```python
from build123d import *

# Parameters (mm, degrees)
SKETCH1_W           = 239
SKETCH1_H           = 85.4
BOSS_EXTRUDE1_DEPTH = 5
SKETCH2_R           = 1.58
CUT_EXTRUDE1_DEPTH  = 254.848695092
CUT_EXTRUDE2_DEPTH  = 254.848695092
SKETCH4_R           = 2.5
SKETCH4_W           = 50
SKETCH4_H           = 15
SKETCH4_W_2         = 19.5
SKETCH4_H_2         = 14
CUT_EXTRUDE3_DEPTH  = 254.848695092
SKETCH5_W           = 5
SKETCH5_H           = 85.4
BOSS_EXTRUDE2_DEPTH = 3


with BuildPart() as part:
    # Sketch1 → Boss-Extrude1 (new body)
    with BuildSketch(Plane.XY):
        with Locations((119.5, 42.7)):
            Rectangle(SKETCH1_W, SKETCH1_H)
    extrude(amount=BOSS_EXTRUDE1_DEPTH)

    # Sketch2 → Cut-Extrude1 (cut, through all)
    with BuildSketch(Plane.XY.offset(5)):
        with Locations((30, 30)):
            Circle(SKETCH2_R)
        with Locations((54.99, 30)):
            Circle(SKETCH2_R)
        with Locations((94.99, 30)):
            Circle(SKETCH2_R)
        with Locations((70, 30)):
            Circle(SKETCH2_R)
        with Locations((134.99, 30)):
            Circle(SKETCH2_R)
        with Locations((110, 30)):
            Circle(SKETCH2_R)
        with Locations((94.99, 50)):
            Circle(SKETCH2_R)
        with Locations((70, 50)):
            Circle(SKETCH2_R)
        with Locations((134.99, 50)):
            Circle(SKETCH2_R)
        with Locations((110, 50)):
            Circle(SKETCH2_R)
        with Locations((94.99, 70)):
            Circle(SKETCH2_R)
        with Locations((70, 70)):
            Circle(SKETCH2_R)
        with Locations((134.99, 70)):
            Circle(SKETCH2_R)
        with Locations((110, 70)):
            Circle(SKETCH2_R)
        with Locations((54.99, 50)):
            Circle(SKETCH2_R)
        with Locations((30, 50)):
            Circle(SKETCH2_R)
        with Locations((54.99, 70)):
            Circle(SKETCH2_R)
        with Locations((30, 70)):
            Circle(SKETCH2_R)
    extrude(amount=-CUT_EXTRUDE1_DEPTH, mode=Mode.SUBTRACT)

    # Sketch3 → Cut-Extrude2 (cut, through all)
    with BuildSketch(Plane.XY.offset(5)):
        with BuildLine():
            Line((31.5267187, 33.043828447), (32.799320889, 24.771914224))
            ThreePointArc((32.799320889, 24.771914224), (33.305182132, 23.861551788), (34.281878435, 23.5))
            Line((34.281878435, 23.5), (50.708121565, 23.5))
            ThreePointArc((50.708121565, 23.5), (51.684817868, 23.861551788), (52.190679111, 24.771914224))
            Line((52.190679111, 24.771914224), (53.4632813, 33.043828447))
            ThreePointArc((53.4632813, 33.043828447), (52.775062631, 35.453392605), (50.498166207, 36.5))
            Line((50.498166207, 36.5), (34.491833793, 36.5))
            ThreePointArc((34.491833793, 36.5), (32.214937369, 35.453392605), (31.5267187, 33.043828447))
        make_face()
        with BuildLine():
            Line((71.5267187, 33.043828447), (72.799320889, 24.771914224))
            ThreePointArc((72.799320889, 24.771914224), (73.305182132, 23.861551788), (74.281878435, 23.5))
            Line((74.281878435, 23.5), (90.708121565, 23.5))
            ThreePointArc((90.708121565, 23.5), (91.684817868, 23.861551788), (92.190679111, 24.771914224))
            Line((92.190679111, 24.771914224), (93.4632813, 33.043828447))
            ThreePointArc((93.4632813, 33.043828447), (92.775062631, 35.453392605), (90.498166207, 36.5))
            Line((90.498166207, 36.5), (74.491833793, 36.5))
            ThreePointArc((74.491833793, 36.5), (72.214937369, 35.453392605), (71.5267187, 33.043828447))
        make_face()
        with BuildLine():
            Line((111.5267187, 33.043828447), (112.799320889, 24.771914224))
            ThreePointArc((112.799320889, 24.771914224), (113.305182132, 23.861551788), (114.281878435, 23.5))
            Line((114.281878435, 23.5), (130.708121565, 23.5))
            ThreePointArc((130.708121565, 23.5), (131.684817868, 23.861551788), (132.190679111, 24.771914224))
            Line((132.190679111, 24.771914224), (133.4632813, 33.043828447))
            ThreePointArc((133.4632813, 33.043828447), (132.775062631, 35.453392605), (130.498166207, 36.5))
            Line((130.498166207, 36.5), (114.491833793, 36.5))
            ThreePointArc((114.491833793, 36.5), (112.214937369, 35.453392605), (111.5267187, 33.043828447))
        make_face()
        with BuildLine():
            Line((71.5267187, 53.043828447), (72.799320889, 44.771914224))
            ThreePointArc((72.799320889, 44.771914224), (73.305182132, 43.861551788), (74.281878435, 43.5))
            Line((74.281878435, 43.5), (90.708121565, 43.5))
            ThreePointArc((90.708121565, 43.5), (91.684817868, 43.861551788), (92.190679111, 44.771914224))
            Line((92.190679111, 44.771914224), (93.4632813, 53.043828447))
            ThreePointArc((93.4632813, 53.043828447), (92.775062631, 55.453392605), (90.498166207, 56.5))
            Line((90.498166207, 56.5), (74.491833793, 56.5))
            ThreePointArc((74.491833793, 56.5), (72.214937369, 55.453392605), (71.5267187, 53.043828447))
        make_face()
        with BuildLine():
            Line((111.5267187, 53.043828447), (112.799320889, 44.771914224))
            ThreePointArc((112.799320889, 44.771914224), (113.305182132, 43.861551788), (114.281878435, 43.5))
            Line((114.281878435, 43.5), (130.708121565, 43.5))
            ThreePointArc((130.708121565, 43.5), (131.684817868, 43.861551788), (132.190679111, 44.771914224))
            Line((132.190679111, 44.771914224), (133.4632813, 53.043828447))
            ThreePointArc((133.4632813, 53.043828447), (132.775062631, 55.453392605), (130.498166207, 56.5))
            Line((130.498166207, 56.5), (114.491833793, 56.5))
            ThreePointArc((114.491833793, 56.5), (112.214937369, 55.453392605), (111.5267187, 53.043828447))
        make_face()
        with BuildLine():
            Line((71.5267187, 73.043828447), (72.799320889, 64.771914224))
            ThreePointArc((72.799320889, 64.771914224), (73.305182132, 63.861551788), (74.281878435, 63.5))
            Line((74.281878435, 63.5), (90.708121565, 63.5))
            ThreePointArc((90.708121565, 63.5), (91.684817868, 63.861551788), (92.190679111, 64.771914224))
            Line((92.190679111, 64.771914224), (93.4632813, 73.043828447))
            ThreePointArc((93.4632813, 73.043828447), (92.775062631, 75.453392605), (90.498166207, 76.5))
            Line((90.498166207, 76.5), (74.491833793, 76.5))
            ThreePointArc((74.491833793, 76.5), (72.214937369, 75.453392605), (71.5267187, 73.043828447))
        make_face()
        with BuildLine():
            Line((111.5267187, 73.043828447), (112.799320889, 64.771914224))
            ThreePointArc((112.799320889, 64.771914224), (113.305182132, 63.861551788), (114.281878435, 63.5))
            Line((114.281878435, 63.5), (130.708121565, 63.5))
            ThreePointArc((130.708121565, 63.5), (131.684817868, 63.861551788), (132.190679111, 64.771914224))
            Line((132.190679111, 64.771914224), (133.4632813, 73.043828447))
            ThreePointArc((133.4632813, 73.043828447), (132.775062631, 75.453392605), (130.498166207, 76.5))
            Line((130.498166207, 76.5), (114.491833793, 76.5))
            ThreePointArc((114.491833793, 76.5), (112.214937369, 75.453392605), (111.5267187, 73.043828447))
        make_face()
        with BuildLine():
            Line((31.5267187, 53.043828447), (32.799320889, 44.771914224))
            ThreePointArc((32.799320889, 44.771914224), (33.305182132, 43.861551788), (34.281878435, 43.5))
            Line((34.281878435, 43.5), (50.708121565, 43.5))
            ThreePointArc((50.708121565, 43.5), (51.684817868, 43.861551788), (52.190679111, 44.771914224))
            Line((52.190679111, 44.771914224), (53.4632813, 53.043828447))
            ThreePointArc((53.4632813, 53.043828447), (52.775062631, 55.453392605), (50.498166207, 56.5))
            Line((50.498166207, 56.5), (34.491833793, 56.5))
            ThreePointArc((34.491833793, 56.5), (32.214937369, 55.453392605), (31.5267187, 53.043828447))
        make_face()
        with BuildLine():
            Line((31.5267187, 73.043828447), (32.799320889, 64.771914224))
            ThreePointArc((32.799320889, 64.771914224), (33.305182132, 63.861551788), (34.281878435, 63.5))
            Line((34.281878435, 63.5), (50.708121565, 63.5))
            ThreePointArc((50.708121565, 63.5), (51.684817868, 63.861551788), (52.190679111, 64.771914224))
            Line((52.190679111, 64.771914224), (53.4632813, 73.043828447))
            ThreePointArc((53.4632813, 73.043828447), (52.775062631, 75.453392605), (50.498166207, 76.5))
            Line((50.498166207, 76.5), (34.491833793, 76.5))
            ThreePointArc((34.491833793, 76.5), (32.214937369, 75.453392605), (31.5267187, 73.043828447))
        make_face()
    extrude(amount=-CUT_EXTRUDE2_DEPTH, mode=Mode.SUBTRACT)

    # Sketch4 → Cut-Extrude3 (cut, through all)
    with BuildSketch(Plane.XY.offset(5)):
        with Locations((188.25, 49.4)):
            Circle(SKETCH4_R)
        with Locations((204, 7.5)):
            Rectangle(SKETCH4_W, SKETCH4_H)
        with Locations((188.25, 65.9)):
            Rectangle(SKETCH4_W_2, SKETCH4_H_2)
    extrude(amount=-CUT_EXTRUDE3_DEPTH, mode=Mode.SUBTRACT)

    # Sketch5 → Boss-Extrude2 (add)
    with BuildSketch(Plane.ZY):
        with Locations((2.5, 42.7)):
            Rectangle(SKETCH5_W, SKETCH5_H)
    extrude(amount=BOSS_EXTRUDE2_DEPTH)


solid = part.part
```
Geometry: final body of the model. Coordinates: model frame, mm. A direction names the side the tool comes from. Give positions to 0.01 mm unless a question says otherwise; leave off trailing zeros. Loops run counter-clockwise (first coordinate to the right, second up) from the corner with the lowest first, then second, coordinate; pieces in that order, holes last. Notation, with made-up numbers: (10, -8.5) -> (42, -8.5) arc R5 ccw to (42, -4.5) -> close; hole circle Ø10 at (64, -34.5). An arc over 180 degrees is marked (long way). Use one line per item in the form item = value.
Item 1: Section query C-C on x = 125. Output: boundary loops of the cut face in (y, z).
A:
outline = (0, 0) -> (23.5, 0) -> (23.5, 5) -> (0, 5) -> close; (36.5, 0) -> (43.5, 0) -> (43.5, 5) -> (36.5, 5) -> close; (56.5, 0) -> (63.5, 0) -> (63.5, 5) -> (56.5, 5) -> close; (76.5, 0) -> (85.4, 0) -> (85.4, 5) -> (76.5, 5) -> close
Item 2: Access query for faces 3 (the face through (204, 15, 3)), 4 (the face through (178.5, 66, 3)). Directions: +Z, -Z, +X, -X, +Y, -Y. A direction counts if a zero-diameter tool reaches every point of the face in a straight line with its end or side. Return the directions, or none.
A:
face_3 = +Z, -Z, -Y
face_4 = +Z, -Z
Item 3: Line query: probe 1 along Y at (x, z) = (88, 4.4); probe 2 along Y at (x, z) = (94.99, 2.25); probe 3 along X at (y, z) = (14, 3.75). Output: solid intervals per line, ascending.
A:
probe_1 = 0 to 23.5, 36.5 to 43.5, 56.5 to 63.5, 76.5 to 85.4
probe_2 = 0 to 28.42, 31.58 to 48.42, 51.58 to 68.42, 71.58 to 85.4
probe_3 = -3 to 179, 229 to 239
Item 4: Section query A-A on x = 183.5. Output: boundary loops of the cut face in (y, z).
A:
outline = (15, 0) -> (58.9, 0) -> (58.9, 5) -> (15, 5) -> close; (72.9, 0) -> (85.4, 0) -> (85.4, 5) -> (72.9, 5) -> close
Item 5: Section query D-D on x = 220.5. Output: boundary loops of the cut face in (y, z).
A:
outline = (15, 0) -> (85.4, 0) -> (85.4, 5) -> (15, 5) -> close
Item 6: Section query B-B on y = 6. Output: boundary loops of the cut face in (x, z), and give its area (3 significant figures).
A:
outline = (-3, 0) -> (179, 0) -> (179, 5) -> (-3, 5) -> close; (229, 0) -> (239, 0) -> (239, 5) -> (229, 5) -> close
area = 960 mm^2
Item 7: Pin query (flat end, axial travel): P1, Ø3, axis at x = 70, y = 70, coming from the -Z side. Return the tip coordinate at first contact, or that it passes through.
A:
P1 = through
Item 8: Draft query along X for faces 1 (the face through (32.154, 48.966, 2.535)), 2 (the face through (120, 85.4, 2)). Return one class per face: pulls with the +X half, pulls with the -X half, needs draft (parallel to the pull), parting line crosses it, or undercut.
A:
face_1 = undercut
face_2 = needs draft
